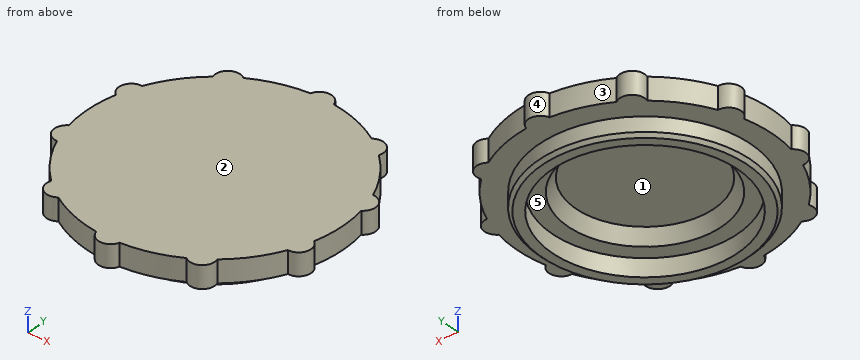
from build123d import *

# Parameters (mm, degrees)
F3_R            = 1.4097
F4_DEPTH        = 2.54
F4_COPIES_COUNT = 10
F5_SIZE         = 0.381


# Not quite as in the source:
# - a pattern or mirror of a feature is missing from the dataset's text; its kind, count and spacing are read off the source's solid


with BuildPart() as f2:
    # F1 (on Front) → F2 (revolve)
    with BuildSketch(Plane.XZ):
        Polygon((-14.605, 0), (-12.0904, 0), (-12.0904, -2.032), (-10.5791, -2.032), (-10.5791, 0), (-8.763, 0), (-7.874, 1.524), (0, 1.524), (0, 2.54), (-14.605, 2.54), align=None)
    revolve(axis=Axis((0, 0, -1.27), (0, 0, -1)))

    # F3 (on face) → F4 (join, through all)
    with BuildSketch(Plane.XY.offset(2.54)):
        with Locations((0, 14.1607994729)):
            Circle(F3_R)
    f4 = extrude(amount=-F4_DEPTH)

    # F4_copies: F4 ×10 about axis
    f4_copies_axis = Axis((0, 0, 0), (0, 0, 1))
    for i in range(1, F4_COPIES_COUNT):
        add(f4.rotate(f4_copies_axis, i * 360 / F4_COPIES_COUNT))

    # F5
    f5_edges = [f2.edges().sort_by_distance(p)[0] for p in [
        (12.0904, 0, -2.032),
    ]]
    chamfer(f5_edges, length=F5_SIZE)


solid = f2.part
Geometry check sheet. Reference: the model listing, model coordinates, mm. Face numbers are marked on the shaded views. A direction names the side the tool comes from. Give positions to 0.01 mm unless a question says otherwise; leave off trailing zeros. Write each loop counter-clockwise with the first axis right and the second up, starting at its lowest first coordinate (ties: lowest second). Pieces come first, ordered by that corner, then holes. Notation, with made-up numbers: M 10,45.25 L 56,45.25 A15 cw 56,67.25 Z; hole C -36.5,88 d10. An arc over 180 degrees is marked long. One line per question, with ' | ' between items.
1. Cross-section at C-C (z = 0.95). Enter the section's corners in (x, y) (1 decimal), plus the area to 3 significant figures.
Ans:
outline: M -14.2,-3.2 A1.4 ccw -13.4,-5.8 A14.6 ccw -9.6,-11 A1.4 ccw -7.4,-12.6 A14.6 ccw -1.4,-14.5 A1.4 ccw 1.4,-14.5 A14.6 ccw 7.4,-12.6 A1.4 ccw 9.6,-11 A14.6 ccw 13.4,-5.8 A1.4 ccw 14.2,-3.2 A14.6 ccw 14.2,3.2 A1.4 ccw 13.4,5.8 A14.6 ccw 9.6,11 A1.4 ccw 7.4,12.6 A14.6 ccw 1.4,14.5 A1.4 ccw -1.4,14.5 A14.6 ccw -7.4,12.6 A1.4 ccw -9.6,11 A14.6 ccw -13.4,5.8 A1.4 ccw -14.2,3.2 A14.6 ccw Z; hole C 0,0 d16.4 | area: 478 mm2
2. Cross-section at B-B (x = 0). Enter the section's corners in (y, z), plus the area to 3 significant figures.
Ans:
outline: M -15.57,0 L -12.09,0 L -12.09,-1.65 L -11.71,-2.03 L -10.58,-2.03 L -10.58,0 L -8.76,0 L -7.87,1.52 L 7.87,1.52 L 8.76,0 L 10.58,0 L 10.58,-2.03 L 11.71,-2.03 L 12.09,-1.65 L 12.09,0 L 15.57,0 L 15.57,2.54 L -15.57,2.54 Z | area: 59.7 mm2
3. Set-up check for the marked faces 4 and 5: record each of +Z, -Z, +X, -X, +Y, -Y from which the full face is reachable in a straight line by a thin tool's end or side.
Ans:
face 4: +Z, -Z, +Y | face 5: -Z
4. Mould release check, pull along Y, two halves, no side actions. Record for the marked faces 1, 2 and 3: released by +Y, released by -Y, zero draft, split by the parting line, or undercut.
Ans:
face 1: undercut | face 2: zero draft | face 3: released by +Y
5. Scan lines: line 1 along Y through (x, z) = (0, -1); line 2 along Z through (x, y) = (-1.25, -6); line 3 along Z through (x, y) = (-0.25, 13). Record each from-to range of solid material in increasing order. Write a range as from..to.
Ans:
line 1: -12.09..-10.58, 10.58..12.09 | line 2: 1.52..2.54 | line 3: 0..2.54
6. Cross-section at A-A (y = 0). Enter the section's corners in (x, z) (3 decimals), plus the area to 3 significant figures.
Ans:
outline: M -14.605,0 L -12.09,0 L -12.09,-1.651 L -11.709,-2.032 L -10.579,-2.032 L -10.579,0 L -8.763,0 L -7.874,1.524 L 7.874,1.524 L 8.763,0 L 10.579,0 L 10.579,-2.032 L 11.709,-2.032 L 12.09,-1.651 L 12.09,0 L 14.605,0 L 14.605,2.54 L -14.605,2.54 Z | area: 54.8 mm2
7. Gauge pin test, flat ends, axial feed: pin 1 (2 mm diameter, centred on y = 10.5, z = 2, fed in from +X); pin 2 (8 mm diameter, centred on x = 0.5, y = 0, fed in from -Z). Record the tip position at first contact, or that the pin passes through.
Ans:
pin 1: x = 11.09 | pin 2: z = 1.52
